Build history of the part. All positions in model axes, mm. Give positions to 0.01 mm unless a question says otherwise; leave off trailing zeros. Order: outer loops, then holes, each group sorted by start corner. A loop starts at its lowest first (then second) coordinate and runs counter-clockwise, first axis right, second up. Notation, with made-up numbers: (89, 63.5) - (112, 63.5) arc R10 ccw to (112, 81.5) - close; hole circle Ø8 at (-34.75, 29.25). An arc over 180 degrees is marked (long way). Write each question's results on one line, items separated by ' | '. Start each with the question number.
1) Drop flat-ended pins along their axis: pin 1 Ø0.6 at (y, z) = (-2.5, 17.5) entering from -X; pin 2 Ø3 at (x, y) = (0, 0) entering from -Z; pin 3 Ø5 at (x, z) = (24.5, 29) entering from +Y. Give the stop position or say it passes through.
2) Drill centre lines: line 1 along X through (y, z) = (0, 36.75); line 2 along Z through (x, y) = (2, 2). Where is each one in solid material? Low to high. Write a range as from..to.
3) Cut at C-C on x = 25.5. List the corners of the cut face in (y, z).
4) Cut at B-B on z = 32. List the corners of the cut face in (x, y).
5) Cut at A-A on y = 0. List the corners of the cut face in (x, z).
from build123d import *

# Parameters (mm, degrees)
SKETCH_1_R          = 2
EXTRUDE_1_DEPTH     = 40
SKETCH_2_W          = 10.776638496
SKETCH_2_H          = 20
CUT_EXTRUDE_2_DEPTH = 20


with BuildPart() as part:
    # Эскиз1 → Вытянуть1 (new body)
    with BuildSketch(Plane.XY):
        with BuildLine():
            Line((2.828427125, -1), (32.828427125, -1))
            Line((32.828427125, -1), (32.828427125, -3))
            Line((32.828427125, -3), (0, -3))
            ThreePointArc((0, -3), (-1.732050808, 2.449489743), (2.828427125, -1))
        make_face()
        Circle(SKETCH_1_R, mode=Mode.SUBTRACT)
    extrude(amount=EXTRUDE_1_DEPTH)

    # Эскиз2 → Вытянуть2 (cut, symmetric)
    with BuildSketch(Plane(origin=(0, 0, 0), x_dir=(1, 0, 0), z_dir=(0, 1, 0))):
        with Locations((-0.445273779, -20)):
            Rectangle(SKETCH_2_W, SKETCH_2_H)
    extrude(amount=CUT_EXTRUDE_2_DEPTH, both=True, mode=Mode.SUBTRACT)


solid = part.part
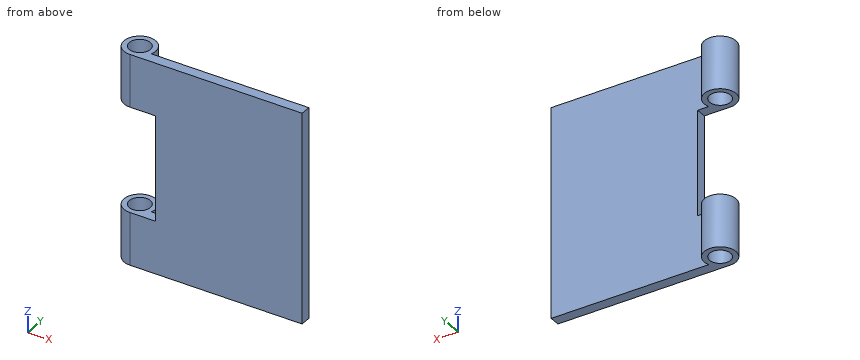
Results:
1) pin 1: x = 4.94 | pin 2: through | pin 3: y = -1
2) line 1: -3..-2, 2..3 | line 2: 0..10, 30..40
3) outline: (-3, 0) - (-1, 0) - (-1, 40) - (-3, 40) - close
4) outline: (0, -3) - (32.83, -3) - (32.83, -1) - (2.83, -1) arc R3 ccw (long way) to start; hole circle Ø4 at (0, 0)
5) outline: (-3, 0) - (-2, 0) - (-2, 10) - (-3, 10) - close; (-3, 30) - (-2, 30) - (-2, 40) - (-3, 40) - close; (2, 0) - (3, 0) - (3, 10) - (2, 10) - close; (2, 30) - (3, 30) - (3, 40) - (2, 40) - close
